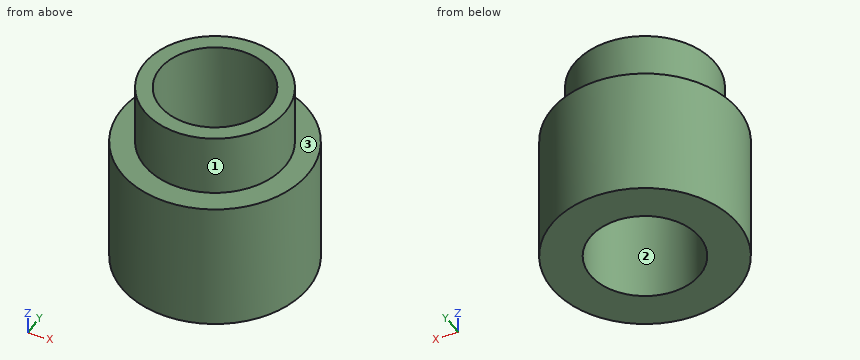
```python
from build123d import *

# Parameters (mm, degrees)
F0_R     = 4.5
F1_DEPTH = 6.35
F2_R     = 3.4
F3_DEPTH = 3
F4_D     = 5.3


with BuildPart() as f1:
    # F0 (on Top) → F1 (new body)
    with BuildSketch(Plane.XY):
        Circle(F0_R)
    extrude(amount=F1_DEPTH)

    # F2 (on face) → F3 (join)
    with BuildSketch(Plane.XY.offset(6.35)):
        Circle(F2_R)
    extrude(amount=F3_DEPTH)

    # F4 (through all)
    with Locations(Plane(origin=(0, 0, 0), x_dir=(1, 0, 0), z_dir=(0, 0, -1))):
        with Locations((0, 0)):
            Hole(F4_D / 2)


solid = f1.part
```
Source: CAD feature listing. Evaluate the final solid. Frame: model axes, mm. Face numbers are marked on the shaded views. Coordinates: 2 decimals unless noted, no trailing zeros. Loops run counter-clockwise (first coordinate to the right, second up) from the corner with the lowest first, then second, coordinate; pieces in that order, holes last. Notation, with made-up numbers: M -22,3 L -11,3 A12 cw -11,25 Z; hole C 72.25,-32 d10. An arc over 180 degrees is marked long. Use a Markdown table: item, result. Add a question column.
Q1. Section query D-D, the plane z = 8. Return loops of the section in (x, y).
Q2. Draft query along X for the marked faces 1, 2 and 3. Return one class per face: pulls with the +X half, pulls with the -X half, needs draft (parallel to the pull), parting line crosses it, or undercut.
Q3. Material intervals for L1, parallel to X at y = 2.25, z = 4.75; L2, parallel to Y at x = 0, z = 3; L3, parallel to Y at x = 2, z = 4, sorted ascending.
Q4. Section query C-C, the plane z = 3.75. Return loops of the section in (x, y).
Q5. Section query A-A, the plane y = 0. Return loops of the section in (x, z).
Q6. First-contact query: pin 1 (1 mm diameter, centred on y = 2, z = 3, fed in from -X). Flat tip, straight axial feed; report the tip coordinate or a pass-through.
Result:
| question | item | result |
|---|---|---|
| 1 | outline | C 0,0 d6.8; hole C 0,0 d5.3 |
| 2 | face 1 | parting line crosses it |
| 2 | face 2 | undercut |
| 2 | face 3 | needs draft |
| 3 | L1 | x = -3.9 to -1.4, 1.4 to 3.9 |
| 3 | L2 | y = -4.5 to -2.65, 2.65 to 4.5 |
| 3 | L3 | y = -4.03 to -1.74, 1.74 to 4.03 |
| 4 | outline | C 0,0 d9; hole C 0,0 d5.3 |
| 5 | outline | M -4.5,0 L -2.65,0 L -2.65,9.35 L -3.4,9.35 L -3.4,6.35 L -4.5,6.35 Z; M 2.65,0 L 4.5,0 L 4.5,6.35 L 3.4,6.35 L 3.4,9.35 L 2.65,9.35 Z |
| 6 | pin 1 | stops at x = -4.24 |
